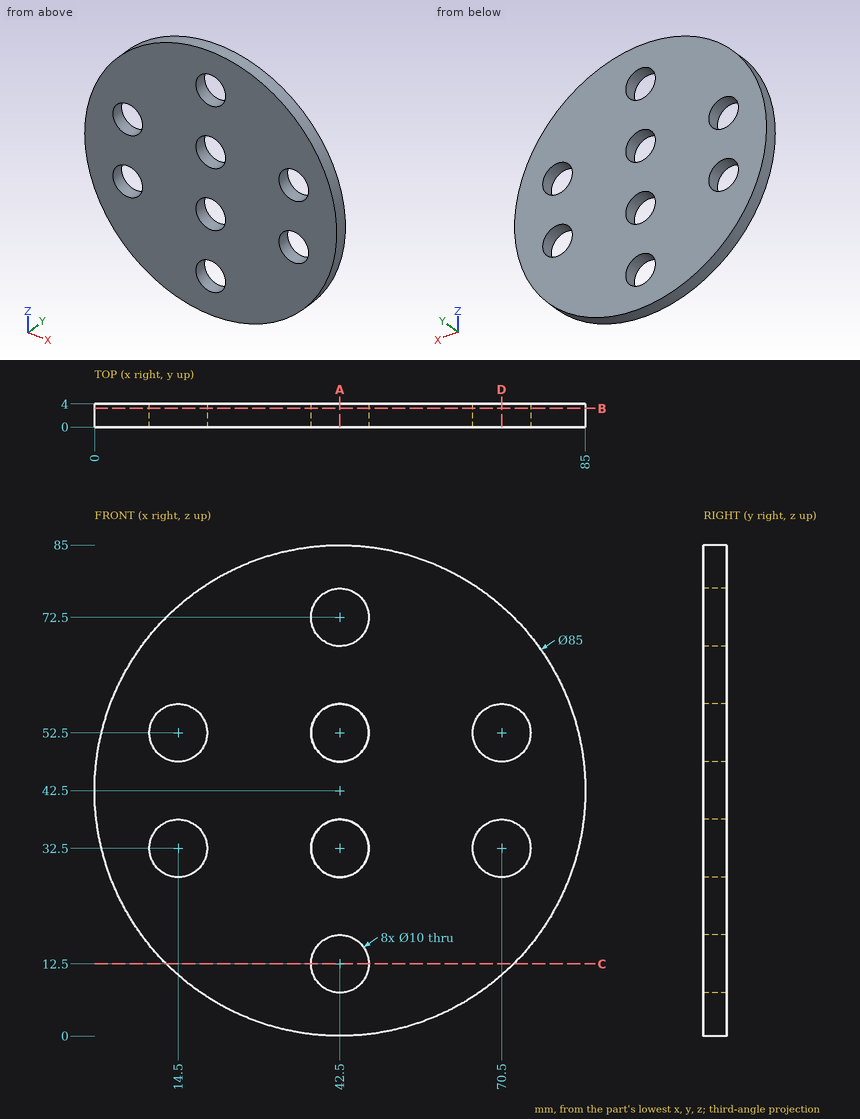
The drawing under review shows one solid part. Ordinate dimensions are in mm from its lowest x, y, z. Round coordinates to 2 decimals unless told otherwise and drop trailing zeros. Loops run counter-clockwise (first coordinate to the right, second up) from the corner with the lowest first, then second, coordinate; pieces in that order, holes last. Notation, with made-up numbers: (21, 61) -> (75, 61) arc R19 cw to (75, 70) -> close; hole circle Ø2 at (66, 47.5). An arc over 180 degrees is marked (long way). Answer in a Markdown table with one row per item.
1) Consider section A-A, the plane x = 42.5. Write out the cut boundary in (y, z), plus the area to 3 significant figures.
Taken from the geometry:
| item | result |
|---|---|
| outline | (0, 0) -> (4, 0) -> (4, 7.5) -> (0, 7.5) -> close; (0, 17.5) -> (4, 17.5) -> (4, 27.5) -> (0, 27.5) -> close; (0, 37.5) -> (4, 37.5) -> (4, 47.5) -> (0, 47.5) -> close; (0, 57.5) -> (4, 57.5) -> (4, 67.5) -> (0, 67.5) -> close; (0, 77.5) -> (4, 77.5) -> (4, 85) -> (0, 85) -> close |
| area | 180 mm² |
2) Consider section D-D, the plane x = 70.5. Write out the cut boundary in (y, z), plus the area to 3 significant figures.
Taken from the geometry:
| item | result |
|---|---|
| outline | (0, 10.53) -> (4, 10.53) -> (4, 27.5) -> (0, 27.5) -> close; (0, 37.5) -> (4, 37.5) -> (4, 47.5) -> (0, 47.5) -> close; (0, 57.5) -> (4, 57.5) -> (4, 74.47) -> (0, 74.47) -> close |
| area | 176 mm² |
3) Consider section B-B, the plane y = 3.25. Count the separate pieces of the cut face and the enclosed holes in it, plus the area to 3 significant figures.
Taken from the geometry:
| item | result |
|---|---|
| separate pieces | 1 |
| enclosed holes | 8 |
| area | 5,050 mm² |
4) Wall thickness on line 1 along Z through (x, y) = (42.5, 2.7); line 2 along Z through (x, y) = (72, 0.3); line 3 along Z through (x, y) = (75, 2.4): over which ranges is each line inside the solid? List them lowest first.
Taken from the geometry:
| item | result |
|---|---|
| line 1 | z = 0 to 7.5, 17.5 to 27.5, 37.5 to 47.5, 57.5 to 67.5, 77.5 to 85 |
| line 2 | z = 11.91 to 27.73, 37.27 to 47.73, 57.27 to 73.09 |
| line 3 | z = 15.11 to 30.32, 34.68 to 50.32, 54.68 to 69.89 |
5) Consider section C-C, the plane z = 12.5. Write out the cut boundary in (x, y).
Taken from the geometry:
| item | result |
|---|---|
| outline | (12.4, 0) -> (37.5, 0) -> (37.5, 4) -> (12.4, 4) -> close; (47.5, 0) -> (72.6, 0) -> (72.6, 4) -> (47.5, 4) -> close |
